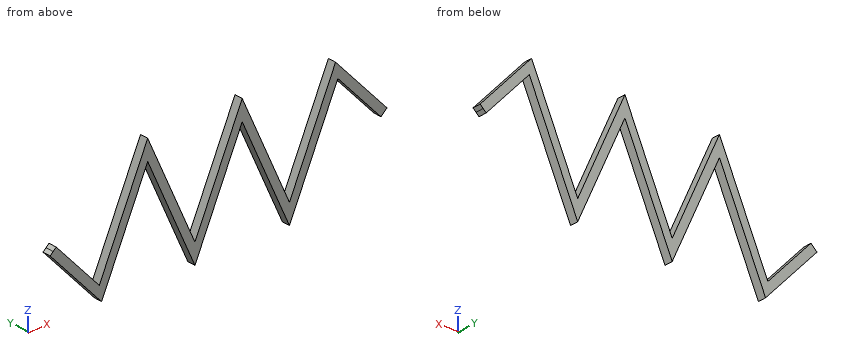
```python
from build123d import *

# Parameters (mm, degrees)
BOSS_EXTRUDE1_DEPTH = 2


with BuildPart() as part:
    # Sketch1 → Boss-Extrude1 (new body)
    with BuildSketch(Plane(origin=(0, 0, 0), x_dir=(1, 0, 0), z_dir=(0, 1, 0))):
        Polygon((-93.922283941, 0.667291311), (-93.177487119, 0), (-81.530301229, 13), (-69.883115339, -13), (-58.235929449, 13), (-46.588743559, -13), (-34.941557669, 13), (-23.29437178, -13), (-11.64718589, 0), (-12.391982712, 0.667291311), (-23.011418731, -11.185586247), (-34.941557669, 15.446049526), (-46.588743559, -10.553950474), (-58.235929449, 15.446049526), (-69.883115339, -10.553950474), (-81.24734818, 14.814413753), align=None)
        Polygon((-81.530301229, 13), (-93.177487119, 0), (-92.432690296, -0.667291311), (-81.813254277, 11.185586247), (-69.883115339, -15.446049526), (-58.235929449, 10.553950474), (-46.588743559, -15.446049526), (-34.941557669, 10.553950474), (-23.577324828, -14.814413753), (-10.902389067, -0.667291311), (-11.64718589, 0), (-23.29437178, -13), (-34.941557669, 13), (-46.588743559, -13), (-58.235929449, 13), (-69.883115339, -13), align=None)
    extrude(amount=BOSS_EXTRUDE1_DEPTH)


solid = part.part
```
The model under review builds one solid part; all positions refer to its coordinate system, in mm. Coordinates: 2 decimals unless noted, no trailing zeros. Write each loop counter-clockwise with the first axis right and the second up, starting at its lowest first coordinate (ties: lowest second). Pieces come first, ordered by that corner, then holes. Notation, with made-up numbers: (72, 79) - (111, 79) arc R32 ccw to (111, 116) - close; hole circle Ø4 at (-23, 82.25). An arc over 180 degrees is marked (long way). Answer in a Markdown table with one row per item. Add a question column.
Q1. Consider section C-C on y = 1.6. Give the boundary of the cut face in (x, z), then the cut area to 3 significant figures.
Q2. To check wall thickness, follow line 1 along X through (y, z) = (0.5, 4); line 2 along X through (y, z) = (1.6, 3); line 3 along X through (y, z) = (0.5, 13.5). State the ranges of each line that lie inside material, in increasing order. Write a range as from..to.
Q3. Consider section B-B on z = 13.5. Give the boundary of the cut face in (x, y), then the cut area to 3 significant figures.
Q4. Clearance check with a flat-ended pin moving along its axis: pin 1 (1 mm diameter, centred on x = -43.5, y = 1.5, fed in from -Z). State where the tip first meets the part, or that it passes through.
Q5. Consider section D-D on x = -65. Give the boundary of the cut face in (y, z).
Q6. Consider section A-A on z = 6. Give the boundary of the cut face in (x, y), then the cut area to 3 significant figures.
Answers below:
| question | item | result |
|---|---|---|
| 1 | outline | (-93.92, -0.67) - (-81.25, -14.81) - (-69.88, 10.55) - (-58.24, -15.45) - (-46.59, 10.55) - (-34.94, -15.45) - (-23.01, 11.19) - (-12.39, -0.67) - (-10.9, 0.67) - (-23.58, 14.81) - (-34.94, -10.55) - (-46.59, 15.45) - (-58.24, -10.55) - (-69.88, 15.45) - (-81.81, -11.19) - (-92.43, 0.67) - close |
| 1 | area | 355 mm² |
| 2 | line 1 | -75.01..-72.82, -66.95..-64.76, -51.72..-49.52, -43.65..-41.46, -28.42..-26.23, -16.57..-13.89 |
| 2 | line 2 | -75.46..-73.27, -66.5..-64.31, -52.16..-49.97, -43.2..-41.01, -28.87..-26.68, -15.68..-12.99 |
| 2 | line 3 | -70.75..-69.01, -47.46..-45.72, -24.17..-22.4 |
| 3 | outline | (-70.75, 0) - (-69.01, 0) - (-69.01, 2) - (-70.75, 2) - close; (-47.46, 0) - (-45.72, 0) - (-45.72, 2) - (-47.46, 2) - close; (-24.17, 0) - (-22.4, 0) - (-22.4, 2) - (-24.17, 2) - close |
| 3 | area | 10.5 mm² |
| 4 | pin 1 | z = 2.54 |
| 5 | outline | (0, -0.35) - (2, -0.35) - (2, 4.55) - (0, 4.55) - close |
| 6 | outline | (-74.11, 0) - (-71.92, 0) - (-71.92, 2) - (-74.11, 2) - close; (-67.84, 0) - (-65.65, 0) - (-65.65, 2) - (-67.84, 2) - close; (-50.82, 0) - (-48.63, 0) - (-48.63, 2) - (-50.82, 2) - close; (-44.55, 0) - (-42.36, 0) - (-42.36, 2) - (-44.55, 2) - close; (-27.53, 0) - (-25.33, 0) - (-25.33, 2) - (-27.53, 2) - close; (-18.37, 0) - (-15.68, 0) - (-15.68, 2) - (-18.37, 2) - close |
| 6 | area | 27.3 mm² |
